Read the model definition and answer for the solid it produces. Units are mm, in the model's axes. A direction names the side the tool comes from. Coordinates: 2 decimals unless noted, no trailing zeros. Order: outer loops, then holes, each group sorted by start corner. A loop starts at its lowest first (then second) coordinate and runs counter-clockwise, first axis right, second up. Notation, with made-up numbers: M 55.5,-31 L 84.5,-31 A20 ccw 84.5,6 Z; hole C -25.75,63.25 d9. An arc over 180 degrees is marked long. Put each result on its own line as item: value.
from build123d import *

# Parameters (mm, degrees)
EXTRUDE_1_DEPTH     = 6
SKETCH_2_R          = 2
CUT_EXTRUDE_1_DEPTH = 10
SKETCH_4_R          = 1.5
CUT_EXTRUDE_2_DEPTH = 6
SKETCH_7_R          = 2
SKETCH_7_R_2        = 1.5
CUT_EXTRUDE_3_DEPTH = 6
SKETCH_5_R          = 8.5
EXTRUDE_4_DEPTH     = 11
FILLET_1_R          = 2
SKETCH_8_R          = 7.55
CUT_EXTRUDE_4_DEPTH = 5
SKETCH_9_R          = 2.95
CUT_EXTRUDE_5_DEPTH = 6


with BuildPart() as part:
    # 草图1 → 凸台-拉伸1 (new body)
    with BuildSketch(Plane(origin=(0, 0, 0), x_dir=(0, 0, -1), z_dir=(1, 0, 0))):
        Polygon((-58.108525398, 10), (-58.108525398, -35), (42.059282617, -35), (42.059282617, -30.677521513), (42.059282617, -25.387821403), (52.220185328, 2.502083897), (58.88447221, 20.794388757), (53.88447221, 20.794388757), (8.88447221, 20.794388757), (10.802160114, 26.733589605), (-8.108525398, 26.733589605), (-50.96776046, 26.733589605), align=None)
    extrude(amount=EXTRUDE_1_DEPTH)

    # 草图2 → 切除-拉伸1 (cut)
    with BuildSketch(Plane(origin=(0, 0, 0), x_dir=(0, 0, -1), z_dir=(1, 0, 0))):
        with Locations((6.512667985, -3.171691559)):
            Circle(SKETCH_2_R)
        with Locations((6.512667985, -13.171691559)):
            Circle(SKETCH_2_R)
        with Locations(Location((-42.117332015, -13.171691559, 0), (0, 0, 180))):
            Circle(SKETCH_2_R)
        with Locations(Location((-42.117332015, -3.171691559, 0), (0, 0, 180))):
            Circle(SKETCH_2_R)
        Polygon((-17.802332015, 1.828308441), (-38.302332015, 1.828308441), (-38.302332015, -18.171691559), (-17.802332015, -18.171691559), (2.697667985, -18.171691559), (2.697667985, 1.828308441), align=None)
    extrude(amount=CUT_EXTRUDE_1_DEPTH, mode=Mode.SUBTRACT)

    # 草图4 → 切除-拉伸2 (cut)
    with BuildSketch(Plane(origin=(6, 0, 0), x_dir=(0, 0, -1), z_dir=(1, 0, 0))):
        with Locations((-48.59776046, 4.328308441)):
            Circle(SKETCH_4_R)
        with Locations((48.50223954, 4.328308441)):
            Circle(SKETCH_4_R)
    extrude(amount=-CUT_EXTRUDE_2_DEPTH, mode=Mode.SUBTRACT)

    # 草图7 → 切除-拉伸3 (cut)
    with BuildSketch(Plane(origin=(6, 0, 0), x_dir=(0, 0, -1), z_dir=(1, 0, 0))):
        with Locations((-54.108525398, 6.828308441)):
            Circle(SKETCH_7_R)
        with Locations((35.891474602, -31.171691559)):
            Circle(SKETCH_7_R)
        with Locations((-54.108525398, -31.171691559)):
            Circle(SKETCH_7_R)
        with BuildLine():
            Line((1.03223954, 18.328308441), (-47.59776046, 18.328308441))
            ThreePointArc((-47.59776046, 18.328308441), (-49.09776046, 16.828308441), (-47.59776046, 15.328308441))
            Line((-47.59776046, 15.328308441), (1.03223954, 15.328308441))
            ThreePointArc((1.03223954, 15.328308441), (2.53223954, 16.828308441), (1.03223954, 18.328308441))
        make_face()
        with BuildLine():
            Line((1.03223954, 23.328308441), (-47.59776046, 23.328308441))
            ThreePointArc((-47.59776046, 23.328308441), (-49.09776046, 21.828308441), (-47.59776046, 20.328308441))
            Line((-47.59776046, 20.328308441), (1.03223954, 20.328308441))
            ThreePointArc((1.03223954, 20.328308441), (2.53223954, 21.828308441), (1.03223954, 23.328308441))
        make_face()
        with BuildLine():
            Line((1.03223954, 13.328308441), (-47.59776046, 13.328308441))
            ThreePointArc((-47.59776046, 13.328308441), (-49.09776046, 11.828308441), (-47.59776046, 10.328308441))
            Line((-47.59776046, 10.328308441), (1.03223954, 10.328308441))
            ThreePointArc((1.03223954, 10.328308441), (2.53223954, 11.828308441), (1.03223954, 13.328308441))
        make_face()
        with BuildLine():
            ThreePointArc((18.012667985, -3.171691559), (16.512667985, -1.671691559), (15.012667985, -3.171691559))
            Line((15.012667985, -3.171691559), (15.012667985, -28.171691559))
            ThreePointArc((15.012667985, -28.171691559), (16.512667985, -29.671691559), (18.012667985, -28.171691559))
            Line((18.012667985, -28.171691559), (18.012667985, -3.171691559))
        make_face()
        with BuildLine():
            ThreePointArc((23.012667985, -3.171691559), (21.512667985, -1.671691559), (20.012667985, -3.171691559))
            Line((20.012667985, -3.171691559), (20.012667985, -28.171691559))
            ThreePointArc((20.012667985, -28.171691559), (21.512667985, -29.671691559), (23.012667985, -28.171691559))
            Line((23.012667985, -28.171691559), (23.012667985, -3.171691559))
        make_face()
        with BuildLine():
            ThreePointArc((38.012667985, -3.171691559), (36.512667985, -1.671691559), (35.012667985, -3.171691559))
            Line((35.012667985, -3.171691559), (35.012667985, -23.171691559))
            ThreePointArc((35.012667985, -23.171691559), (36.512667985, -24.671691559), (38.012667985, -23.171691559))
            Line((38.012667985, -23.171691559), (38.012667985, -3.171691559))
        make_face()
        with BuildLine():
            ThreePointArc((28.012667985, -3.171691559), (26.512667985, -1.671691559), (25.012667985, -3.171691559))
            Line((25.012667985, -3.171691559), (25.012667985, -23.171691559))
            ThreePointArc((25.012667985, -23.171691559), (26.512667985, -24.671691559), (28.012667985, -23.171691559))
            Line((28.012667985, -23.171691559), (28.012667985, -3.171691559))
        make_face()
        with BuildLine():
            ThreePointArc((33.012667985, -3.171691559), (31.512667985, -1.671691559), (30.012667985, -3.171691559))
            Line((30.012667985, -3.171691559), (30.012667985, -23.171691559))
            ThreePointArc((30.012667985, -23.171691559), (31.512667985, -24.671691559), (33.012667985, -23.171691559))
            Line((33.012667985, -23.171691559), (33.012667985, -3.171691559))
        make_face()
        with Locations((-47.59776046, -28.171691559)):
            Circle(SKETCH_7_R_2)
        with Locations((29.50223954, -28.171691559)):
            Circle(SKETCH_7_R_2)
    extrude(amount=-CUT_EXTRUDE_3_DEPTH, mode=Mode.SUBTRACT)

    # 草图5 → 凸台-拉伸4 (add)
    with BuildSketch(Plane(origin=(6, 0, 0), x_dir=(0, 0, -1), z_dir=(1, 0, 0))):
        with Locations((35, 10)):
            Circle(SKETCH_5_R)
    extrude(amount=-EXTRUDE_4_DEPTH)

    # 圆角1
    fillet_1_edges = [part.edges().sort_by_distance(p)[0] for p in [
        (3, 10, 58.108525398),
        (3, 26.733589605, 50.96776046),
        (3, 26.733589605, -10.802160114),
        (3, 20.794388757, -8.88447221),
        (3, 20.794388757, -58.88447221),
        (3, -25.387821403, -42.059282617),
        (3, -35, -42.059282617),
        (3, -35, 58.108525398),
    ]]
    fillet(fillet_1_edges, radius=FILLET_1_R)

    # 草图8 → 切除-拉伸4 (cut)
    with BuildSketch(Plane.ZY.offset(5)):
        with Locations((-35, 10)):
            Circle(SKETCH_8_R)
    extrude(amount=-CUT_EXTRUDE_4_DEPTH, mode=Mode.SUBTRACT)

    # 草图9 → 切除-拉伸5 (cut)
    with BuildSketch(Plane.ZY):
        with Locations((-35, 10)):
            Circle(SKETCH_9_R)
    extrude(amount=-CUT_EXTRUDE_5_DEPTH, mode=Mode.SUBTRACT)


solid = part.part
Q1. Find section B-B on x = -2.5. Write down the section's boundary in (y, z).
Answers below:
outline: C 10,-35 d17; hole C 10,-35 d15.1
Q2. For a pull along Z with two mould halves and no side action, classify faces 3 (the face through (3, -35, 9)), 4 (the face through (2.96, -13.26, 40.12)), 5 (the face through (3.04, -34.43, -41.46)) as +Z half, -Z half, draft (parallel to the pull), parting line (faces both ways), or undercut.
Answers below:
face 3: draft
face 4: undercut
face 5: -Z half
Q3. A tool of negligible diameter and unlimited length cuts with its end or side. For faces 1 (the face through (3.04, -29.67, -16.48)), 2 (the face through (-2.535, 5.406, -40.991)), from which of +Z, -Z, +X, -X, +Y, -Y can it reach the whole face along a straight path? Write none if from no direction.
Answers below:
face 1: +X, -X
face 2: -X
Q4. Find section C-C on z = -6. Write down the section's boundary in (x, y).
Answers below:
outline: M 0,-35 L 6,-35 L 6,-15.1 L 0,-15.1 Z; M 0,-11.24 L 6,-11.24 L 6,-5.1 L 0,-5.1 Z; M 0,-1.24 L 6,-1.24 L 6,26.73 L 0,26.73 Z
Q5. Find section D-D on x = 3.25. Give the number of separate pieces and of enclosed holes in the cut face, plus the area to 3 significant figures.
Answers below:
separate pieces: 1
enclosed holes: 21
area: 4,530 mm^2
Q6. Consider line 1 along Y through (x, z) = (2.5, 20); line 2 along Y through (x, z) = (2.75, 46); line 3 along Z through (x, y) = (1, -23.5). Determine where each line is inside the solid, lowest interval first.
Answers below:
line 1: y = -35 to -18.17, 1.83 to 10.33, 13.33 to 15.33, 18.33 to 20.33, 23.33 to 26.73
line 2: y = -35 to 10.33, 13.33 to 15.33, 18.33 to 20.33, 23.33 to 26.73
line 3: z = -42.75 to -37.98, -35.05 to -32.98, -30.05 to -27.98, -25.05 to -23.01, -20.01 to -18.01, -15.01 to 58.11
Q7. Given pin 1 (1.8 mm diameter, centred on x = 2, y = -15.5, fed in from -Z); pin 2 (6.5 mm diameter, centred on y = -13.17, z = 42.12, fed in from -X); pin 3 (1.8 mm diameter, centred on x = 2.5, y = -18.5, fed in from -Z), each flat-ended and moving along its own axis, determine where each tip first touches the part or whether it passes through.
Answers below:
pin 1: stops at z = -45.99
pin 2: stops at x = 0
pin 3: stops at z = -44.9
Q8. Find section A-A on z = 7. Write down the section's boundary in (x, y).
Answers below:
outline: M 0,-35 L 6,-35 L 6,-18.17 L 0,-18.17 Z; M 0,1.83 L 6,1.83 L 6,10.33 L 0,10.33 Z; M 0,13.33 L 6,13.33 L 6,15.33 L 0,15.33 Z; M 0,18.33 L 6,18.33 L 6,20.33 L 0,20.33 Z; M 0,23.33 L 6,23.33 L 6,26.73 L 0,26.73 Z
